```python
from build123d import *

# Parameters (mm, degrees)
REVOLVE1_ANGLE      = 90.0000000000002
SKETCH5_R           = 2.5000000000000013
CUT_EXTRUDE3_DEPTH  = 13.000000000000002
SKETCH6_R           = 2.5000000000000004
CUT_EXTRUDE4_DEPTH  = 13.000000000000002
SKETCH7_R           = 2.5000000000000013
CUT_EXTRUDE5_DEPTH  = 13.000000000000002
CUT_REVOLVE14_ANGLE = 90.0000000000002
CUT_EXTRUDE20_DEPTH = 0.9999999999999974
CUT_EXTRUDE24_DEPTH = 1
CUT_EXTRUDE25_DEPTH = 1


with BuildPart() as part:
    # Sketch4 → Revolve1 (revolve)
    with BuildSketch(Plane(origin=(0, 0, 0), x_dir=(1, 0, 0), z_dir=(0, 1, 0))):
        with BuildLine():
            Line((0, 0), (15, 0))
            ThreePointArc((15, 0), (10.606601717798213, 10.606601717798211), (0, 15))
            Line((0, 15), (0, 0))
        make_face()
    revolve(axis=Axis((0, 0, 0), (1, 0, 0)), revolution_arc=REVOLVE1_ANGLE)

    # Sketch5 → Cut-Extrude3 (cut)
    with BuildSketch(Plane.XY):
        with Locations((3, 3)):
            Circle(SKETCH5_R)
    extrude(amount=-CUT_EXTRUDE3_DEPTH, mode=Mode.SUBTRACT)

    # Sketch6 → Cut-Extrude4 (cut)
    with BuildSketch(Plane.ZY):
        with Locations((-3, 3)):
            Circle(SKETCH6_R)
    extrude(amount=-CUT_EXTRUDE4_DEPTH, mode=Mode.SUBTRACT)

    # Sketch7 → Cut-Extrude5 (cut)
    with BuildSketch(Plane.XZ):
        with Locations(Location((3, -3, 0), (0, 0, 270))):
            Circle(SKETCH7_R)
    extrude(amount=-CUT_EXTRUDE5_DEPTH, mode=Mode.SUBTRACT)

    # Sketch8 → Cut-Revolve14 (revolve, cut)
    with BuildSketch(Plane.XY):
        with BuildLine():
            ThreePointArc((4.767766952966368, 4.767766952966372), (2.580296881351315, 6.229387725907349), (0, 6.742640687119288))
            Line((0, 6.742640687119287), (0, 0))
            Line((0, 0), (6.742640687119288, 4.1e-16))
            ThreePointArc((6.742640687119288, 1.52e-15), (6.229387725907348, 2.5802968813513187), (4.767766952966368, 4.767766952966372))
        make_face()
        with BuildLine():
            ThreePointArc((5.500000000000002, 2.9999999999999996), (0.6903011687217822, 2.043291419087274), (4.767766952966367, 4.767766952966372))
            ThreePointArc((4.767766952966367, 4.767766952966372), (5.309698831278217, 3.9567085809127267), (5.500000000000002, 3))
        make_face(mode=Mode.SUBTRACT)
    revolve(axis=Axis((0, 0, 0), (0, 1, 3.49e-15)), revolution_arc=CUT_REVOLVE14_ANGLE, mode=Mode.SUBTRACT)

    # Sketch9 → Cut-Extrude20 (cut)
    with BuildSketch(Plane.XY):
        with BuildLine():
            ThreePointArc((11.6081867662439, 9.499999999999998), (10.606601717798215, 10.60660171779821), (9.500000000000005, 11.608186766243897))
            Line((9.500000000000005, 11.608186766243898), (11.608186766243902, 9.499999999999998))
        make_face()
        with BuildLine():
            Line((11.608186766243902, 9.499999999999998), (9.500000000000005, 11.608186766243898))
            Line((9.500000000000005, 11.608186766243898), (3.5956903599630037, 5.703877126206902))
            ThreePointArc((3.5956903599630796, 5.703877126206793), (4.207841503717712, 5.268517183723248), (4.767766952966372, 4.7677669529663715))
            ThreePointArc((4.767766952966372, 4.7677669529663715), (5.268517183723248, 4.207841503717712), (5.703877126206793, 3.5956903599630796))
            Line((5.703877126206905, 3.5956903599630046), (11.608186766243902, 9.499999999999998))
        make_face()
        with BuildLine():
            ThreePointArc((4.767766952966372, 4.7677669529663715), (4.207841503717712, 5.268517183723248), (3.5956903599630796, 5.703877126206793))
            Line((3.5956903599630037, 5.703877126206902), (-1.0540933831219501, 1.0540933831219519))
            Line((-1.0540933831219503, 1.054093383121952), (1.0540933831219486, -1.0540933831219486))
            Line((1.0540933831219483, -1.0540933831219483), (5.703877126206905, 3.5956903599630046))
            ThreePointArc((5.703877126206793, 3.5956903599630796), (5.268517183723248, 4.207841503717712), (4.767766952966372, 4.7677669529663715))
        make_face()
    extrude(amount=-CUT_EXTRUDE20_DEPTH, mode=Mode.SUBTRACT)

    # Sketch10 → Cut-Extrude24 (cut)
    with BuildSketch(Plane.ZY):
        with BuildLine():
            Line((-8.999999999999977, 11.999999999999961), (-11.999999999999998, 9.000000000000002))
            Line((-11.999999999999998, 9.000000000000002), (-6.025660362620837, 3.025660362620844))
            ThreePointArc((-6.025660362621033, 3.0256603626207323), (-5.466557614006139, 3.947144700710623), (-4.76776695296637, 4.767766952966371))
            ThreePointArc((-4.767766952966371, 4.767766952966371), (-3.947144700710626, 5.466557614006138), (-3.0256603626207372, 6.025660362621032))
            Line((-3.02566036262085, 6.025660362620837), (-8.999999999999977, 11.999999999999961))
        make_face()
        with BuildLine():
            ThreePointArc((-9.000000000000004, 11.999999999999996), (-10.606601717798211, 10.606601717798213), (-12, 9))
            Line((-11.999999999999998, 9.000000000000002), (-8.999999999999977, 11.999999999999961))
        make_face()
        with BuildLine():
            ThreePointArc((-4.76776695296637, 4.767766952966371), (-5.466557614006139, 3.947144700710623), (-6.025660362621033, 3.0256603626207323))
            Line((-6.025660362620837, 3.025660362620844), (-1.4999999999999947, -1.4999999999999947))
            Line((-1.4999999999999944, -1.4999999999999944), (1.499999999999994, 1.4999999999999944))
            Line((1.4999999999999947, 1.4999999999999947), (-3.02566036262085, 6.025660362620837))
            ThreePointArc((-3.0256603626207372, 6.025660362621032), (-3.947144700710626, 5.466557614006138), (-4.767766952966371, 4.767766952966371))
        make_face()
    extrude(amount=-CUT_EXTRUDE24_DEPTH, mode=Mode.SUBTRACT)

    # Sketch11 → Cut-Extrude25 (cut)
    with BuildSketch(Plane.XZ):
        with BuildLine():
            Line((11.999999999999996, -9.000000000000002), (9.000000000000002, -11.999999999999998))
            ThreePointArc((8.999999999999996, -12.000000000000002), (10.60660171779821, -10.606601717798215), (11.999999999999998, -9.000000000000002))
        make_face()
        with BuildLine():
            Line((3.0256603626208403, -6.025660362620841), (9.000000000000002, -11.999999999999998))
            Line((9.000000000000002, -11.999999999999998), (11.999999999999996, -9.000000000000002))
            Line((11.999999999999996, -9.000000000000002), (6.02566036262084, -3.0256603626208403))
            ThreePointArc((6.025660362621034, -3.025660362620727), (5.466557614006142, -3.9471447007106204), (4.767766952966371, -4.767766952966369))
            ThreePointArc((4.7677669529663715, -4.767766952966372), (3.9471447007106226, -5.466557614006144), (3.0256603626207275, -6.025660362621036))
        make_face()
        with BuildLine():
            Line((-1.5000000000000036, -1.5), (3.0256603626208403, -6.025660362620841))
            ThreePointArc((3.0256603626207275, -6.025660362621036), (3.9471447007106226, -5.466557614006144), (4.7677669529663715, -4.767766952966372))
            ThreePointArc((4.767766952966371, -4.767766952966369), (5.466557614006142, -3.9471447007106204), (6.025660362621034, -3.025660362620727))
            Line((6.02566036262084, -3.0256603626208403), (1.5, 1.5000000000000036))
            Line((1.4999999999999996, 1.5000000000000036), (-1.500000000000003, -1.4999999999999996))
        make_face()
    extrude(amount=-CUT_EXTRUDE25_DEPTH, mode=Mode.SUBTRACT)


solid = part.part
```
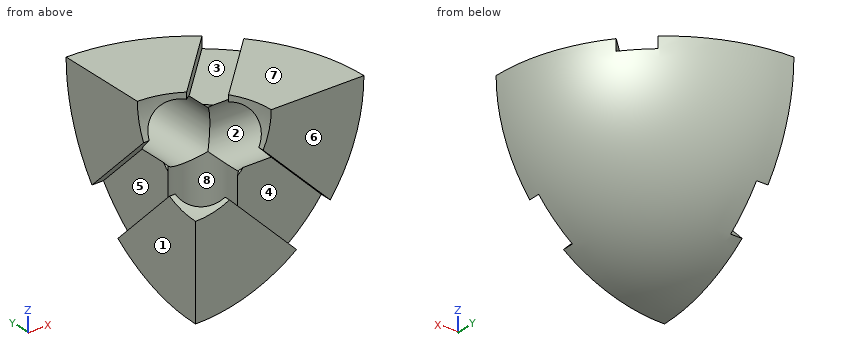
Here's how the part is built. I have some questions about the finished solid (model axes, mm). Face numbers are marked on the shaded views. A direction names the side the tool comes from. Round coordinates to 2 decimals unless told otherwise and drop trailing zeros. Order: outer loops, then holes, each group sorted by start corner. A loop starts at its lowest first (then second) coordinate and runs counter-clockwise, first axis right, second up. Notation, with made-up numbers: (-10.75, 17.25) -> (-6.75, 17.25) arc R17 ccw to (-6.75, 21.25) -> close; hole circle Ø9 at (19.5, 58.25). An arc over 180 degrees is marked (long way). Use a Markdown table: item, result. Add a question column.
(1) If we mould it in two halves opening along Y, with no side actions, what happens to the marked faces 5, 6, 7 and 8? For each: released by +Y, released by -Y, zero draft, split by the parting line, or undercut.
(2) Suppose I cut it at C-C, the plane z = -4. Please give me the cut outline in (x, y), and give its area (3 significant figures).
(3) Suppose I cut it at A-A, the plane x = 6.25. Please give me the cut outline in (y, z), and give its area (3 significant figures).
(4) Suppose I cut it at B-B, the plane y = 11. Please give me the cut outline in (x, z).
(5) Suppose I cut it at D-D, the plane x = 4. Please give me the cut outline in (y, z), and give its area (3 significant figures).
(6) For pin 1 Ø4 at (x, y) = (5, 6.5) entering from -Z; pin 2 Ø1.5 at (x, z) = (2.5, -2.5) entering from -Y; pin 3 Ø3 at (x, y) = (6.5, 1.5) entering from -Z; pin 4 Ø3 at (y, z) = (12.5, -11.5) entering from -X, each with a flat end and sliding along its axis, tell me the tip position at first contact or that it passes through.
(7) I need wall thicknesses on line 1 along X through (y, z) = (3, -9.5); line 2 along Y through (x, z) = (10.5, -3); line 3 along Z through (x, y) = (3, 11). Which ranges of each line are inside material? Lowest first, please.
(8) For the marked faces 1, 2, 3 and 4, which set-ups out of +Z, -Z, +X, -X, +Y, -Y let a thin tool reach every point of the face, with its end or its side?
Verdict:
| question | item | result |
|---|---|---|
| 1 | face 5 | undercut |
| 1 | face 6 | released by -Y |
| 1 | face 7 | zero draft |
| 1 | face 8 | undercut |
| 2 | outline | (0, 7) -> (0.71, 7) -> (0.71, 13) -> (5.29, 13) -> (5.29, 5.29) -> (13, 5.29) -> (13, 0.71) -> (7, 0.71) -> (7, 0) -> (14.46, 0) arc R14.46 ccw to (0, 14.46) -> close |
| 2 | area | 63.1 mm2 |
| 3 | outline | (0, -13.64) arc R13.64 ccw to (13.64, 0) -> (8.36, 0) -> (8.36, -1) -> (4.5, -1) arc R2.5 cw (long way) to (1, -4.5) -> (1, -9.25) -> (0, -9.25) -> close; (0, -3.25) -> (0.51, -3.25) arc R2.5 cw to (0.56, -2.47) arc R2.53 cw to (0, -2.53) -> close; (2.47, -0.56) arc R2.5 cw to (4.14, -0.78) -> (4.14, 0) -> (2.53, 0) arc R2.53 cw to start |
| 3 | area | 113 mm2 |
| 4 | outline | (0, -8) -> (1, -8) -> (1, -10.15) arc R10.2 ccw to (10.15, -1) -> (8.89, -1) -> (8.89, 0) -> (0, 0) -> close; hole circle Ø5 at (3, -3) |
| 5 | outline | (0, -14.46) arc R14.46 ccw to (14.46, 0) -> (6.11, 0) -> (6.11, -0.71) -> (13, -0.71) -> (13, -5.29) -> (5.29, -5.29) -> (5.29, -13) -> (0.71, -13) -> (0.71, -7) -> (0, -7) -> close |
| 5 | area | 63.7 mm2 |
| 6 | pin 1 | z = -13.66 |
| 6 | pin 2 | y = 13 |
| 6 | pin 3 | z = -14.08 |
| 6 | pin 4 | through |
| 7 | line 1 | 0 to 0.5, 5.5 to 11.21 |
| 7 | line 2 | 0 to 0.5, 5.5 to 10.28 |
| 7 | line 3 | -9.75 to -5.5, -0.5 to 0 |
| 8 | face 1 | +Z, -Z, -X, +Y, -Y |
| 8 | face 2 | -X |
| 8 | face 3 | +Z |
| 8 | face 4 | -Y |
